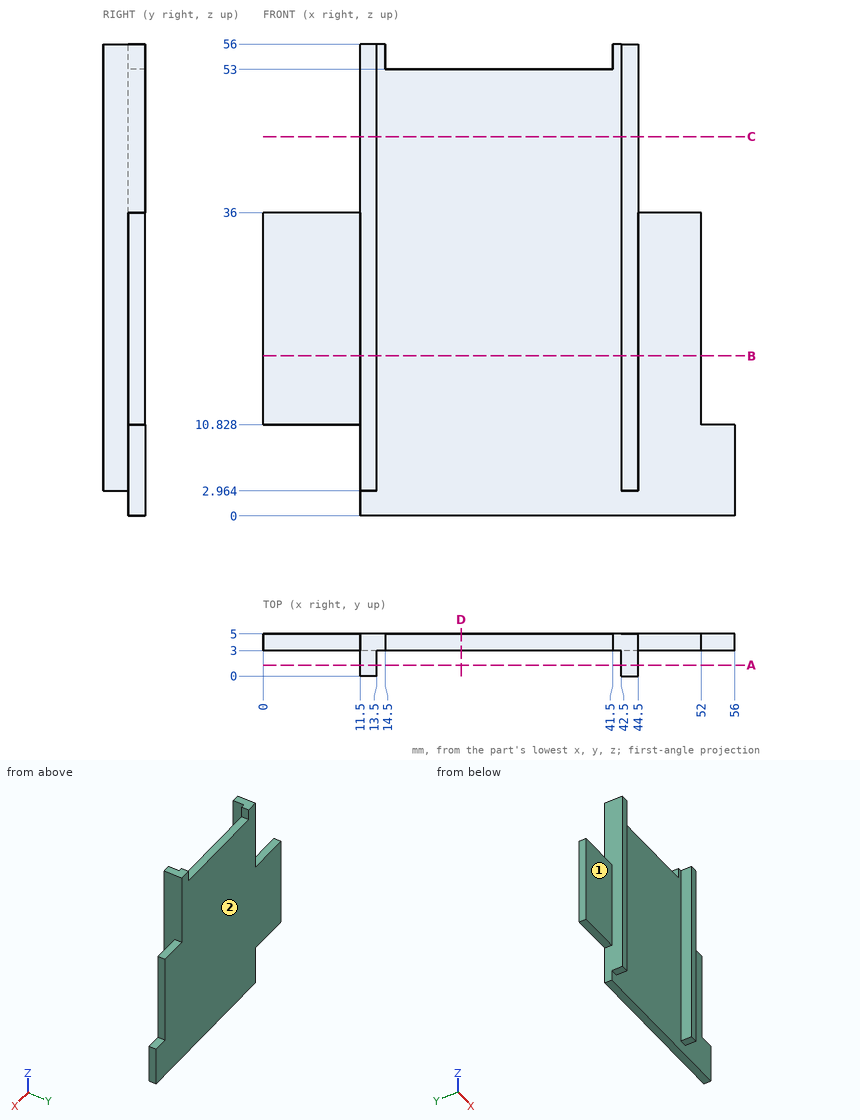
Print and shaded views of the part. All mm, measured from the part's lowest x, y and z. A direction names the side the tool comes from. Give positions to 0.01 mm unless a question says otherwise; leave off trailing zeros. Loops run counter-clockwise (first coordinate to the right, second up) from the corner with the lowest first, then second, coordinate; pieces in that order, holes last.
1) Saw through at C-C (z = 45). Write the cut outline in (x, y).
2) Tool access for the marked faces 1 and 2: list every direction of +Z, -Z, +X, -X, +Y, -Y with a clear straight run to the whole face (end or side of a thin tool).
3) Saw through at A-A (y = 1.3). Write the cut outline in (x, z), plus the area to 3 significant figures.
4) Wall check: line 1 (X direction, y = 1.9, z = 16); line 2 (Y direction, x = 27.5, z = 28); line 3 (Z direction, x = 6, y = 4.65). Give the ranges that are in metal, low to high.
5) Flat gauge pins, fed straight in: pin 1 Ø3.5 at (x, z) = (4.5, 29) entering from -Y; pin 2 Ø1 at (x, y) = (7.5, 4) entering from -Z; pin 3 Ø2.5 at (y, z) = (1.5, 34) entering from -X; pin 4 Ø6 at (x, z) = (41, 49) entering from -Y. Where does each tip first touch, or does it go through?
6) Saw through at D-D (x = 23.5). Write the cut outline in (y, z), plus the area to 3 significant figures.
7) Saw through at B-B (z = 19). Write the cut outline in (x, y), plus the area to 3 significant figures.
Answer block:
1. outline: (11.5, 0) - (13.5, 0) - (13.5, 3) - (42.5, 3) - (42.5, 0) - (44.5, 0) - (44.5, 5) - (11.5, 5) - close
2. face 1: +Z, -Z, -X, -Y
2. face 2: +Z, -Z, +X, -X, +Y
3. outline: (11.5, 2.96) - (13.5, 2.96) - (13.5, 56) - (11.5, 56) - close; (42.5, 2.96) - (44.5, 2.96) - (44.5, 56) - (42.5, 56) - close
3. area: 212 mm2
4. line 1: x = 11.5 to 13.5, 42.5 to 44.5
4. line 2: y = 3 to 5
4. line 3: z = 10.83 to 36
5. pin 1: stops at y = 3
5. pin 2: stops at z = 10.83
5. pin 3: stops at x = 11.5
5. pin 4: stops at y = 0
6. outline: (3, 0) - (5, 0) - (5, 53) - (3, 53) - close
6. area: 106 mm2
7. outline: (0, 3) - (11.5, 3) - (11.5, 0) - (13.5, 0) - (13.5, 3) - (42.5, 3) - (42.5, 0) - (44.5, 0) - (44.5, 3) - (52, 3) - (52, 5) - (0, 5) - close
7. area: 116 mm2
